```python
from build123d import *

# Parameters (mm, degrees)
SKETCH1_W           = 30
SKETCH1_H           = 34
BOSS_EXTRUDE1_DEPTH = 5
FILLET2_R           = 5
SKETCH10_R          = 1.75
CUT_EXTRUDE7_DEPTH  = 6
SKETCH11_W          = 3.733694592
SKETCH11_H          = 11
CUT_EXTRUDE8_DEPTH  = 1.2
DRAFT1_ANGLE        = 20
FILLET3_R           = 0.4


with BuildPart() as part:
    # Sketch1 → Boss-Extrude1 (new body)
    with BuildSketch(Plane.XZ.offset(5)):
        Rectangle(SKETCH1_W, SKETCH1_H)
    extrude(amount=-BOSS_EXTRUDE1_DEPTH)

    # Fillet2
    fillet2_edges = [part.edges().sort_by_distance(p)[0] for p in [
        (15, -2.5, 17),
        (15, -2.5, -17),
        (-15, -2.5, -17),
        (-15, -2.5, 17),
    ]]
    fillet(fillet2_edges, radius=FILLET2_R)

    # Sketch10 → Cut-Extrude7 (cut, through all)
    with BuildSketch(Plane.XZ.offset(5)):
        with Locations((0, 11.25)):
            Circle(SKETCH10_R)
        with Locations((0, -11.25)):
            Circle(SKETCH10_R)
    extrude(amount=-CUT_EXTRUDE7_DEPTH, mode=Mode.SUBTRACT)

    # Sketch11 → Cut-Extrude8 (cut)
    with BuildSketch(Plane.XZ.offset(5)):
        with Locations((-12.5, 0)):
            Rectangle(SKETCH11_W, SKETCH11_H)
        with Locations((-7.5, 0)):
            Rectangle(SKETCH11_W, SKETCH11_H)
        with Locations((-2.5, 0)):
            Rectangle(SKETCH11_W, SKETCH11_H)
        with Locations((2.5, 0)):
            Rectangle(SKETCH11_W, SKETCH11_H)
        with Locations((7.5, 0)):
            Rectangle(SKETCH11_W, SKETCH11_H)
        with Locations((12.5, 0)):
            Rectangle(SKETCH11_W, SKETCH11_H)
    extrude(amount=-CUT_EXTRUDE8_DEPTH, mode=Mode.SUBTRACT)

    # Draft1
    draft1_faces = [part.faces().sort_by_distance(p)[0] for p in [
        (10.633152704, -4.4, 0),
        (5.633152704, -4.4, 0),
        (0.633152704, -4.4, 0),
        (-4.366847296, -4.4, 0),
        (-9.366847296, -4.4, 0),
        (-14.366847296, -4.4, 0),
        (14.366847296, -4.4, 0),
        (9.366847296, -4.4, 0),
        (4.366847296, -4.4, 0),
        (-0.633152704, -4.4, 0),
        (-5.633152704, -4.4, 0),
        (-10.633152704, -4.4, 0),
    ]]
    draft(draft1_faces, Plane(origin=(0, -5, 0), x_dir=(0, 0, -1), z_dir=(0, -1, 0)), DRAFT1_ANGLE)

    # Fillet3
    fillet3_edges = [part.edges().sort_by_distance(p)[0] for p in [
        (-13.930083015, -3.8, 0),
        (-11.069916985, -3.8, 0),
        (-14.366847296, -5, 0),
        (-10.633152704, -5, 0),
        (-8.930083015, -3.8, 0),
        (-6.069916985, -3.8, 0),
        (-9.366847296, -5, 0),
        (-5.633152704, -5, 0),
        (-3.930083015, -3.8, 0),
        (-1.069916985, -3.8, 0),
        (-4.366847296, -5, 0),
        (-0.633152704, -5, 0),
        (1.069916985, -3.8, 0),
        (3.930083015, -3.8, 0),
        (0.633152704, -5, 0),
        (4.366847296, -5, 0),
        (6.069916985, -3.8, 0),
        (8.930083015, -3.8, 0),
        (5.633152704, -5, 0),
        (9.366847296, -5, 0),
        (11.069916985, -3.8, 0),
        (13.930083015, -3.8, 0),
        (10.633152704, -5, 0),
        (14.366847296, -5, 0),
    ]]
    fillet(fillet3_edges, radius=FILLET3_R)


solid = part.part
```
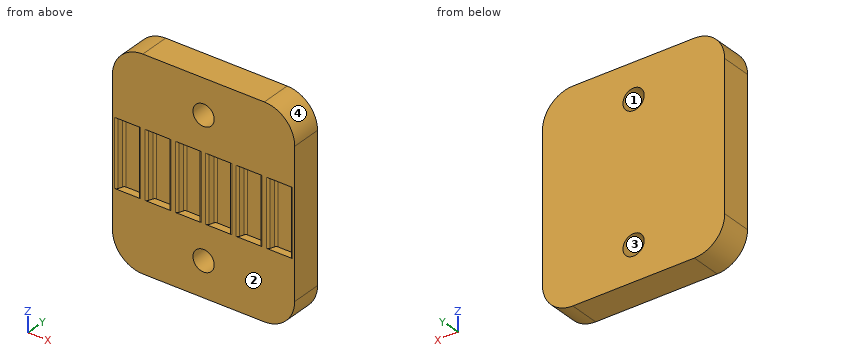
CAD build for the part. Positions are in the model's coordinates, mm. Face numbers are marked on the shaded views. Coordinates: 2 decimals unless noted, no trailing zeros. Order: outer loops, then holes, each group sorted by start corner. A loop starts at its lowest first (then second) coordinate and runs counter-clockwise, first axis right, second up. Notation, with made-up numbers: (72, -37.75) - (78, -37.75) arc R31 ccw to (78, 1.25) - close; hole circle Ø7 at (14.5, 67). An arc over 180 degrees is marked (long way). Use a Markdown table: item, result. Add a question column.
(1) Flat gauge pins, fed straight in: pin 1 (1 mm diameter, centred on x = 13, y = -4.5, fed in from -Z); pin 2 (1.8 mm diameter, centred on x = -2.5, z = -1, fed in from -Y); pin 3 (1.8 mm diameter, centred on x = -7, z = 2, fed in from -Y). Where does each tip first touch, or does it go through?
(2) Saw through at D-D (z = 14). Give the cut face in (x, y), then the cut area to 3 significant figures.
(3) Saw through at B-B (x = -3.25). Give the cut face in (y, z), then the cut area to 3 significant figures.
(4) Pull direction X, two halves, no side cores. Call the marked faces 1, 2, 3 and 4: +X half, -X half, draft (parallel to the pull), parting line (faces both ways), or undercut.
(5) Saw through at A-A (z = -11.25). Give the cut face in (x, y).
(6) Drill centre lines: line 1 along Z through (x, y) = (0, -3.05); line 2 along X through (y, z) = (-1.35, 10.5); line 3 along Z through (x, y) = (10.25, -0.75). Where is each one in solid material? Low to high. Write a range as [from, to].
(7) Saw through at C-C (y = -2.1). Give the cut face in (x, z), then the cut area to 3 significant figures.
Solved:
| question | item | result |
|---|---|---|
| 1 | pin 1 | stops at z = -16.33 |
| 1 | pin 2 | stops at y = -3.8 |
| 1 | pin 3 | stops at y = -3.89 |
| 2 | outline | (-14.58, -5) - (14.58, -5) - (14.58, 0) - (-14.58, 0) - close |
| 2 | area | 146 mm² |
| 3 | outline | (-5, -17) - (0, -17) - (0, 17) - (-5, 17) - (-5, 5.5) - (-3.8, 5.5) - (-3.8, -5.5) - (-5, -5.5) - close |
| 3 | area | 157 mm² |
| 4 | face 1 | undercut |
| 4 | face 2 | draft |
| 4 | face 3 | undercut |
| 4 | face 4 | +X half |
| 5 | outline | (-15, -5) - (-1.75, -5) - (-1.75, 0) - (-15, 0) - close; (1.75, -5) - (15, -5) - (15, 0) - (1.75, 0) - close |
| 6 | line 1 | z = [-17, -13], [-9.5, 9.5], [13, 17] |
| 6 | line 2 | x = [-15, -1.58], [1.58, 15] |
| 6 | line 3 | z = [-16.99, 16.99] |
| 7 | outline | (-15, -12) arc R5 ccw to (-10, -17) - (10, -17) arc R5 ccw to (15, -12) - (15, 12) arc R5 ccw to (10, 17) - (-10, 17) arc R5 ccw to (-15, 12) - close; hole circle Ø3.5 at (0, -11.25); hole circle Ø3.5 at (0, 11.25) |
| 7 | area | 979 mm² |
